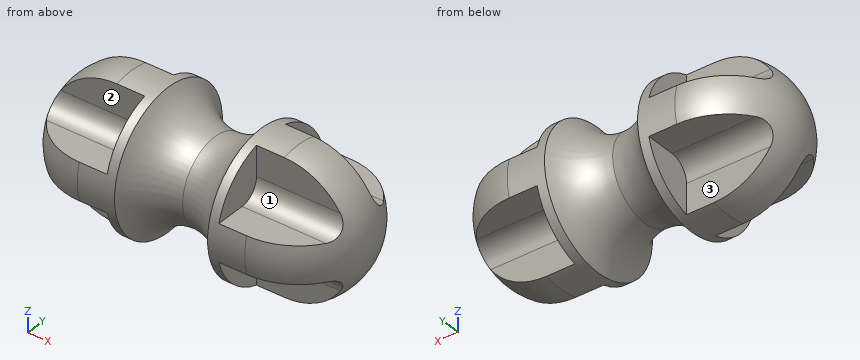
from build123d import *

# Parameters (mm, degrees)
SKETCH_1_W               = 5
SKETCH_1_H               = 37.5
CUT_EXTRUDE_1_DEPTH      = 77.40353395
PATTERN_CIRCULAR_1_COUNT = 4
MIRROR_2_COPY_1_DEPTH    = 77.40353395
MIRROR_2_COPY_2_DEPTH    = 77.40353395
MIRROR_2_COPY_3_DEPTH    = 77.40353395


with BuildPart() as part:
    # 草图1 → 旋转1 (revolve)
    with BuildSketch(Plane(origin=(0, 0, 0), x_dir=(1, 0, 0), z_dir=(0, 1, 0))):
        with BuildLine():
            Line((-82.5, 0), (-30, 0))
            Line((-30, 0), (-30, 37.5))
            Line((-30, 37.5), (-45, 37.5))
            ThreePointArc((-45, 37.5), (-71.516504294, 26.516504294), (-82.5, 0))
        make_face()
        with Locations((-27.5, 18.75)):
            Rectangle(SKETCH_1_W, SKETCH_1_H)
        with BuildLine():
            Line((-25, 0), (0, 0))
            Line((0, 0), (0, 22.5))
            ThreePointArc((0, 22.5), (-14.577379737, 26.537700438), (-25, 37.5))
            Line((-25, 37.5), (-25, 0))
        make_face()
        with BuildLine():
            Line((0, 22.5), (0, 0))
            Line((0, 0), (25, 0))
            Line((25, 0), (25, 37.5))
            ThreePointArc((25, 37.5), (14.577379737, 26.537700438), (0, 22.5))
        make_face()
    revolve_1 = revolve(axis=Axis((0, 0, 0), (-1, 0, 0)))

    # 草图2 → 切除-拉伸1 (cut, through all)
    with BuildSketch(Plane(origin=(-30, 0, 0), x_dir=(0, 0, -1), z_dir=(1, 0, 0))):
        with BuildLine():
            Line((10, 54.755645053), (54.446031679, 54.755645053))
            Line((54.446031679, 54.755645053), (54.446031679, 10))
            Line((54.446031679, 10), (20, 10))
            ThreePointArc((20, 10), (12.928932188, 12.928932188), (10, 20))
            Line((10, 20), (10, 54.755645053))
        make_face()
    cut_extrude_1 = extrude(amount=-CUT_EXTRUDE_1_DEPTH, mode=Mode.SUBTRACT)

    # 阵列(圆周)1: 切除-拉伸1 ×4 about axis
    pattern_circular_1_axis = Axis((0, 0, 0), (1, 0, 0))
    for i in range(1, PATTERN_CIRCULAR_1_COUNT):
        add(cut_extrude_1.rotate(pattern_circular_1_axis, i * 360 / PATTERN_CIRCULAR_1_COUNT), mode=Mode.SUBTRACT)

    # 镜向2: 旋转1, 切除-拉伸1 across plane
    add(revolve_1.mirror(Plane(origin=(0, 0, 0), x_dir=(0, 0, 1), z_dir=(1, 0, 0))))
    add(cut_extrude_1.mirror(Plane(origin=(0, 0, 0), x_dir=(0, 0, 1), z_dir=(1, 0, 0))), mode=Mode.SUBTRACT)

    # 镜向2 copy 1 sketch → 镜向2 copy 1 (cut, through all)
    with BuildSketch(Plane(origin=(30, 0, 0), x_dir=(0, 1, 0), z_dir=(-1, 0, 0))):
        with BuildLine():
            Line((10, -54.755645053), (54.446031679, -54.755645053))
            Line((54.446031679, -54.755645053), (54.446031679, -10))
            Line((54.446031679, -10), (20, -10))
            ThreePointArc((20, -10), (12.928932188, -12.928932188), (10, -20))
            Line((10, -20), (10, -54.755645053))
        make_face()
    extrude(amount=-MIRROR_2_COPY_1_DEPTH, mode=Mode.SUBTRACT)

    # 镜向2 copy 2 sketch → 镜向2 copy 2 (cut, through all)
    with BuildSketch(Plane.ZY.offset(-30)):
        with BuildLine():
            Line((10, -54.755645053), (54.446031679, -54.755645053))
            Line((54.446031679, -54.755645053), (54.446031679, -10))
            Line((54.446031679, -10), (20, -10))
            ThreePointArc((20, -10), (12.928932188, -12.928932188), (10, -20))
            Line((10, -20), (10, -54.755645053))
        make_face()
    extrude(amount=-MIRROR_2_COPY_2_DEPTH, mode=Mode.SUBTRACT)

    # 镜向2 copy 3 sketch → 镜向2 copy 3 (cut, through all)
    with BuildSketch(Plane(origin=(30, 0, 0), x_dir=(0, -1, 0), z_dir=(-1, 0, 0))):
        with BuildLine():
            Line((10, -54.755645053), (54.446031679, -54.755645053))
            Line((54.446031679, -54.755645053), (54.446031679, -10))
            Line((54.446031679, -10), (20, -10))
            ThreePointArc((20, -10), (12.928932188, -12.928932188), (10, -20))
            Line((10, -20), (10, -54.755645053))
        make_face()
    extrude(amount=-MIRROR_2_COPY_3_DEPTH, mode=Mode.SUBTRACT)


solid = part.part
Geometry check sheet. Reference: the model listing, model coordinates, mm. Face numbers are marked on the shaded views. A direction names the side the tool comes from. Coordinates: 2 decimals unless noted, no trailing zeros. Write each loop counter-clockwise with the first axis right and the second up, starting at its lowest first coordinate (ties: lowest second). Pieces come first, ordered by that corner, then holes. Notation, with made-up numbers: (-3, 87.25) -> (42, 87.25) arc R13 ccw to (42, 106.25) -> close; hole circle Ø10 at (10.25, 75). An arc over 180 degrees is marked (long way). One line per question, with ' | ' between items.
1. Thickness scan on probe 1 along Z at (x, y) = (-65.5, -22); probe 2 along X at (y, z) = (-15, -12); probe 3 along X at (y, z) = (-30.5, 4.5). Record the ranges inside material, lowest first. Write a range as from..to.
Answers:
probe 1: z = -10..10 | probe 2: x = -30..30 | probe 3: x = -66.35..-20.07, 20.07..66.35
2. Cross-section at B-B on x = 54.5. Record the cut outline in (y, z), and give its area (3 significant figures).
Answers:
outline: (-34.87, -10) -> (-20, -10) arc R10 cw to (-10, -20) -> (-10, -34.87) arc R36.28 ccw to (10, -34.87) -> (10, -20) arc R10 cw to (20, -10) -> (34.87, -10) arc R36.28 ccw to (34.87, 10) -> (20, 10) arc R10 cw to (10, 20) -> (10, 34.87) arc R36.28 ccw to (-10, 34.87) -> (-10, 20) arc R10 cw to (-20, 10) -> (-34.87, 10) arc R36.28 ccw to start | area: 2,550 mm²
3. Set-up check for the marked faces 1, 2 and 3: record each of +Z, -Z, +X, -X, +Y, -Y from which the full face is reachable in a straight line by a thin tool's end or side.
Answers:
face 1: +Z, +X, -Y | face 2: +Z, -X, -Y | face 3: -Z, -X, +Y
4. Depth check by flat-ended pin: pin 1 Ø13 at (y, z) = (19, -21) entering from +X; pin 2 Ø3 at (y, z) = (18, 11) entering from -X; pin 3 Ø8 at (x, y) = (3, 1.5) entering from -Z. Enter the tip coordinate at first touch or a pass-through.
Answers:
pin 1: stops at x = 30 | pin 2: stops at x = -76.97 | pin 3: stops at z = -23.35
5. Cross-section at A-A on x = -36.5. Record the cut outline in (y, z), and give its area (3 significant figures).
Answers:
outline: (-36.14, -10) -> (-20, -10) arc R10 cw to (-10, -20) -> (-10, -36.14) arc R37.5 ccw to (10, -36.14) -> (10, -20) arc R10 cw to (20, -10) -> (36.14, -10) arc R37.5 ccw to (36.14, 10) -> (20, 10) arc R10 cw to (10, 20) -> (10, 36.14) arc R37.5 ccw to (-10, 36.14) -> (-10, 20) arc R10 cw to (-20, 10) -> (-36.14, 10) arc R37.5 ccw to start | area: 2,650 mm²
6. Cross-section at C-C on x = 28. Record the cut outline in (y, z).
Answers:
outline: circle Ø75 at (0, 0)
7. Cross-section at D-D on x = 11. Record the cut outline in (y, z), and give its area (3 significant figures).
Answers:
outline: circle Ø49.44 at (0, 0) | area: 1,920 mm²
